Autodesk Inventor part; units mm, degrees
ref_plane "YZ Plane" through (0, 0, 0) normal (1, 0, 0) x (0, 1, 0)
ref_plane "XZ Plane" through (0, 0, 0) normal (0, 1, 0) x (-1, 0, 0)
ref_plane "XY Plane" through (0, 0, 0) normal (0, 0, 1) x (1, 0, 0)
sketch "Sketch1" plane through (0, 0, 0) normal (1, 0, 0) x (0, 1, 0)
  line L0 (25, -50) -> (-25, -50)
  line L1 (-25, -50) -> (-25, 50)
  line L2 (-25, 50) -> (25, 50)
  line L3 (25, 50) -> (25, -50)
  line L4 (25, -50) -> (-25, 50) construction
  line L5 (-25, -50) -> (25, 50) construction
  point P0 (0, 0)
  dimension "d0" = 50
  dimension "d1" = 100
extrude "Extrusion1" add sketch "Sketch1" along normal mid plane 559
fillet "Fillet1" radius 4 4 edges at (0, 25, 50) (0, -25, 50) (0, -25, -50) (0, 25, -50)
shell "Shell1" thickness 4 removed faces 2 at (-279.5, -8.3333, -15.3333) at (279.5, -8.3333, -15.3333)
properties part number "MC03-1"
Here's how the part is built. I have some questions about the finished solid (model axes, mm). A direction names the side the tool comes from. Round coordinates to 2 decimals unless told otherwise and drop trailing zeros. Write each loop counter-clockwise with the first axis right and the second up, starting at its lowest first coordinate (ties: lowest second). Pieces come first, ordered by that corner, then holes.
1. Suppose I cut it at A-A (z = 24.5). List the corners of the cut face in (x, y) for me.
2. I need wall thicknesses on L1, parallel to Z at x = 37, y = -19; L2, parallel to Y at x = 33.5, z = 31; L3, parallel to Z at x = 77.5, y = 21.5. Which ranges of each line are inside material? Lowest first, please.
3. Suppose I cut it at C-C (x = -18.5). List the corners of the cut face in (y, z) for me.
4. If we mould it in two halves opening along Y, with no side actions, what happens to faces 1 (the flat face through (-4, -25, -1)), 2 (the flat face through (-4, 0, -46)), 3 (the flat face through (279.5, -22, 4))? For each: released by +Y, released by -Y, zero draft, split by the parting line, or undercut.
5. For faces 4 (the flat face through (-4, 25, 1)), 5 (the flat face through (-4, -21, -1)), which set-ups out of +Z, -Z, +X, -X, +Y, -Y let a thin tool reach every point of the face, with its end or its side?
6. Suppose I cut it at B-B (y = 15). List the corners of the cut face in (x, z) for me, and give its area (3 significant figures).
7. Will this pin go through, and if not, where does the flat tip stop? pin 1 Ø5 at (y, z) = (17.5, -21) entering from -X.
Answer sheet:
1. outline: (-279.5, -25) - (279.5, -25) - (279.5, -21) - (-279.5, -21) - close; (-279.5, 21) - (279.5, 21) - (279.5, 25) - (-279.5, 25) - close
2. L1: z = -50 to -46, 46 to 50
2. L2: y = -25 to -21, 21 to 25
2. L3: z = -49.97 to 49.97
3. outline: (-25, -46) arc R4 ccw to (-21, -50) - (21, -50) arc R4 ccw to (25, -46) - (25, 46) arc R4 ccw to (21, 50) - (-21, 50) arc R4 ccw to (-25, 46) - close; hole (-21, -46) - (21, -46) - (21, 46) - (-21, 46) - close
4. face 1: released by -Y
4. face 2: undercut
4. face 3: zero draft
5. face 4: +Z, -Z, +X, -X, +Y
5. face 5: +X, -X
6. outline: (-279.5, -50) - (279.5, -50) - (279.5, -46) - (-279.5, -46) - close; (-279.5, 46) - (279.5, 46) - (279.5, 50) - (-279.5, 50) - close
6. area: 4,470 mm2
7. pin 1: passes through
